The listing builds one solid part. Answer for the finished solid, in the listing's coordinates (mm). Coordinates: 2 decimals unless noted, no trailing zeros. Order: outer loops, then holes, each group sorted by start corner. A loop starts at its lowest first (then second) coordinate and runs counter-clockwise, first axis right, second up. Notation, with made-up numbers: M 86,16.25 L 93,16.25 A23 cw 93,51.25 Z; hole C 44,16.25 d9. An arc over 180 degrees is marked long. One line per item, written item: value. Start each with the question number.
Q1. The part is cut by section B-B on x = 65. Give the vertices of the cut face in (y, z).
Q2. Determine the mould class of faces 1 (the flat face through (-5, 120, 0)), 2 (the cylindrical face through (151.457, 14.248, 3.131)), 3 (the cylindrical face through (-17.95, 129.77, 3.22)) for opening direction Y: pulls with the +Y half, pulls with the -Y half, needs draft (parallel to the pull), parting line crosses it, or undercut.
Q3. The part is cut by section A-A on y = 88. Give the vertices of the cut face in (x, z).
Q4. Straight lines are drawn through the part: line 1 along Y through (x, z) = (-18, 2.75); line 2 along X through (y, z) = (130, 3); line 3 along Y through (x, z) = (51.5, 3.75). For each, find the intervals that lie inside material, in ascending order. Write a range as [from, to].
Q5. The part is cut by section C-C on z = 4.5. Give the number of separate pieces and of enclosed holes in the cut face, then the cut area to 3 significant figures.
Q6. Each of these flat-tipped pins is pushed along its axis until it touches: pin 1 Ø4.5 at (x, y) = (-18.62, -20.07) entering from +Z; pin 2 Ø3 at (y, z) = (10, 3.5) entering from -X; pin 3 Ø1 at (x, z) = (3, 5.5) entering from +Y; pin 4 Ø1.5 at (x, z) = (75, 2) entering from -Y. Where does it stop, or does it pass through?
```python
from build123d import *

# Parameters (mm, degrees)
SKETCH1_R           = 107.95
SKETCH1_R_2         = 83.82
BOSS_EXTRUDE1_DEPTH = 6.35
SKETCH2_R           = 2.085
SKETCH2_R_2         = 2.413
CUT_EXTRUDE1_DEPTH  = 21.336
SKETCH5_R           = 2.413
CUT_EXTRUDE4_DEPTH  = 6.35


with BuildPart() as part:
    # Sketch1 → Boss-Extrude1 (new body)
    with BuildSketch(Plane.XY):
        with Locations((51.738381467, 55.593319394)):
            Circle(SKETCH1_R)
        with Locations((51.738381467, 55.593319394)):
            Circle(SKETCH1_R_2, mode=Mode.SUBTRACT)
    extrude(amount=BOSS_EXTRUDE1_DEPTH)

    # Sketch2 → Cut-Extrude1 (cut)
    with BuildSketch(Plane(origin=(0, 0, 0), x_dir=(-1, 0, 0), z_dir=(0, 0, -1))):
        with Locations((-0.938381467, -32.39486163)):
            Circle(SKETCH2_R)
        with Locations((-102.538381467, -32.39486163)):
            Circle(SKETCH2_R)
        with Locations((-153.338381467, 55.593319394)):
            Circle(SKETCH2_R)
        with Locations((-102.538381467, 143.581500419)):
            Circle(SKETCH2_R)
        with Locations((-0.938381467, 143.581500419)):
            Circle(SKETCH2_R)
        with Locations((49.861618533, 55.593319394)):
            Circle(SKETCH2_R)
        with Locations((-121.212212689, -20.941506669)):
            Circle(SKETCH2_R_2)
        with Locations((18.615381385, -20.066128285)):
            Circle(SKETCH2_R_2)
    extrude(amount=-CUT_EXTRUDE1_DEPTH, mode=Mode.SUBTRACT)

    # Sketch5 → Cut-Extrude4 (cut)
    with BuildSketch(Plane.XY.offset(6.35)):
        with Locations((122.06341072, 131.252946958)):
            Circle(SKETCH5_R)
        with Locations((-17.430655728, 132.126237322)):
            Circle(SKETCH5_R)
    extrude(amount=-CUT_EXTRUDE4_DEPTH, mode=Mode.SUBTRACT)


solid = part.part
```
Output:
1. outline: M -51.54,0 L -27.17,0 L -27.17,6.35 L -51.54,6.35 Z; M 138.36,0 L 162.73,0 L 162.73,6.35 L 138.36,6.35 Z
2. face 1: needs draft
2. face 2: parting line crosses it
2. face 3: undercut
3. outline: M -51.23,0 L -25.56,0 L -25.56,6.35 L -51.23,6.35 Z; M 129.04,0 L 154.71,0 L 154.71,6.35 L 129.04,6.35 Z
4. line 1: y = [-26.81, -22.4], [-17.73, 9.09], [102.09, 129.78], [134.47, 137.99]
4. line 2: x = [-26.47, -18.57], [-16.29, 13.15], [90.33, 120], [124.13, 129.95]
4. line 3: y = [-52.36, -28.23], [139.41, 163.54]
5. separate pieces: 1
5. enclosed holes: 11
5. area: 14,400 mm^2
6. pin 1: passes through
6. pin 2: stops at x = -46.8
6. pin 3: stops at y = 152.17
6. pin 4: stops at y = -49.98
